```python
from build123d import *

# Parameters (mm, degrees)
SCHIZZO1_W                   = 65
SCHIZZO1_H                   = 80
ESTRUSIONE_ESTRUSIONE3_DEPTH = 20
SCHIZZO4_W                   = 61
SCHIZZO4_H                   = 76
TAGLIO_ESTRUSIONE5_DEPTH     = 18
SCHIZZO6_W                   = 11
SCHIZZO6_H                   = 8.5
TAGLIO_ESTRUSIONE8_DEPTH     = 3
SCHIZZO7_R                   = 5.182753919
ESTRUSIONE_ESTRUSIONE6_DEPTH = 17


with BuildPart() as part:
    # Schizzo1 → Estrusione-Estrusione3 (new body)
    with BuildSketch(Plane.XY):
        with Locations((-250.828848217, 316.320789782)):
            Rectangle(SCHIZZO1_W, SCHIZZO1_H)
    extrude(amount=ESTRUSIONE_ESTRUSIONE3_DEPTH)

    # Schizzo4 → Taglio-Estrusione5 (cut)
    with BuildSketch(Plane(origin=(0, 0, 0), x_dir=(-1, 0, 0), z_dir=(0, 0, -1))):
        with Locations((250.785132486, 316.761133349)):
            Rectangle(SCHIZZO4_W, SCHIZZO4_H)
    extrude(amount=-TAGLIO_ESTRUSIONE5_DEPTH, mode=Mode.SUBTRACT)

    # Schizzo6 → Taglio-Estrusione8 (cut)
    with BuildSketch(Plane(origin=(0, 276.320789782, 0), x_dir=(-1, 0, 0), z_dir=(0, -1, 0))):
        with Locations((254.830379364, -3.404987236)):
            Rectangle(SCHIZZO6_W, SCHIZZO6_H)
    extrude(amount=-TAGLIO_ESTRUSIONE8_DEPTH, mode=Mode.SUBTRACT)

    # Schizzo7 → Estrusione-Estrusione6 (add)
    with BuildSketch(Plane(origin=(0, 0, 18), x_dir=(-1, 0, 0), z_dir=(0, 0, -1))):
        with Locations(Location((251.224275907, 345.746509499, 0), (0, 0, 180))):
            Circle(SCHIZZO7_R)
    extrude(amount=ESTRUSIONE_ESTRUSIONE6_DEPTH)


solid = part.part
```
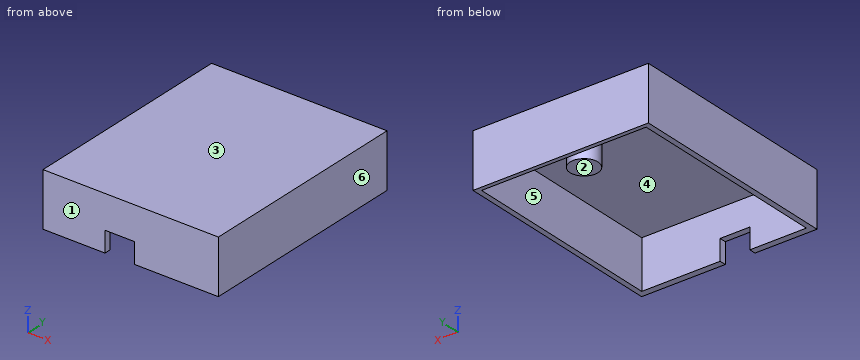
Verification items for the finished model (mm, model axes). Face numbers are marked on the shaded views. A direction names the side the tool comes from. Give positions to 0.01 mm unless a question says otherwise; leave off trailing zeros. Order: outer loops, then holes, each group sorted by start corner. A loop starts at its lowest first (then second) coordinate and runs counter-clockwise, first axis right, second up. Notation, with made-up numbers: (-24, 0) -> (6, 0) arc R21 ccw to (6, 17) -> close; hole circle Ø9 at (43, 22.5). An arc over 180 degrees is marked (long way). Use a Markdown table: item, result.
1) Section check C-C, the plane x = -227.5. Record the boundary of the cut face in (y, z), then the cut area to 3 significant figures.
Results:
| item | result |
|---|---|
| outline | (276.32, 0) -> (278.76, 0) -> (278.76, 18) -> (354.76, 18) -> (354.76, 0) -> (356.32, 0) -> (356.32, 20) -> (276.32, 20) -> close |
| area | 232 mm² |
2) Section check B-B, the plane y = 313. Record the boundary of the cut face in (x, z), then the cut area to 3 significant figures.
Results:
| item | result |
|---|---|
| outline | (-283.33, 0) -> (-281.29, 0) -> (-281.29, 18) -> (-220.29, 18) -> (-220.29, 0) -> (-218.33, 0) -> (-218.33, 20) -> (-283.33, 20) -> close |
| area | 202 mm² |
3) Depth check by flat-ended pin: pin 1 Ø6 at (x, y) = (-243.5, 319.5) entering from -Z; pin 2 Ø0.7 at (x, y) = (-254.5, 277) entering from -Z (3 decimals); pin 3 Ø5 at (x, y) = (-253, 344.5) entering from -Z. Enter the tip coordinate at first touch or a pass-through.
Results:
| item | result |
|---|---|
| pin 1 | z = 18 |
| pin 2 | z = 7.655 |
| pin 3 | z = 1 |
4) Mould release check, pull along X, two halves, no side actions. Record for the marked faces 3, 4, 5 and 6: pulls with the +X half, pulls with the -X half, needs draft (parallel to the pull), parting line crosses it, or undercut.
Results:
| item | result |
|---|---|
| face 3 | needs draft |
| face 4 | undercut |
| face 5 | undercut |
| face 6 | pulls with the +X half |
5) Tool access check on the marked faces 1 and 2. Record the directions out of +Z, -Z, +X, -X, +Y, -Y that give a thin tool (end or side, any length) a straight path to the whole face; none if there is none.
Results:
| item | result |
|---|---|
| face 1 | +Z, -Z, +X, -X, -Y |
| face 2 | -Z |
6) Section check A-A, the plane z = 15. Record the boundary of the cut face in (x, y), then the cut area to 3 significant figures.
Results:
| item | result |
|---|---|
| outline | (-283.33, 276.32) -> (-218.33, 276.32) -> (-218.33, 356.32) -> (-283.33, 356.32) -> close; circle Ø10.37 at (-251.22, 345.75); hole (-281.29, 278.76) -> (-220.29, 278.76) -> (-220.29, 354.76) -> (-281.29, 354.76) -> close |
| area | 648 mm² |
7) Material ranges on probe 1 along Y at (x, z) = (-275.5, 15.5); probe 2 along X at (y, z) = (333, 8.5); probe 3 along Y at (x, z) = (-247, 16.5), recorded low to high.
Results:
| item | result |
|---|---|
| probe 1 | 276.32 to 278.76, 354.76 to 356.32 |
| probe 2 | -283.33 to -281.29, -220.29 to -218.33 |
| probe 3 | 276.32 to 278.76, 342.74 to 348.75, 354.76 to 356.32 |
8) Section check D-D, the plane z = 5.75. Record the boundary of the cut face in (x, y), then the cut area to 3 significant figures.
Results:
| item | result |
|---|---|
| outline | (-283.33, 276.32) -> (-260.33, 276.32) -> (-260.33, 278.76) -> (-281.29, 278.76) -> (-281.29, 354.76) -> (-220.29, 354.76) -> (-220.29, 278.76) -> (-249.33, 278.76) -> (-249.33, 276.32) -> (-218.33, 276.32) -> (-218.33, 356.32) -> (-283.33, 356.32) -> close; circle Ø10.37 at (-251.22, 345.75) |
| area | 622 mm² |
